Input: part model. Units: mm. Frame: model coordinates. A direction names the side the tool comes from. Round coordinates to 2 decimals unless told otherwise and drop trailing zeros. Loops run counter-clockwise (first coordinate to the right, second up) from the corner with the lowest first, then second, coordinate; pieces in that order, holes last. Notation, with made-up numbers: (-18.75, 15.25) - (27.25, 15.25) arc R24 cw to (27.25, 44.25) - close; hole circle Ø11 at (69.25, -11.75). An arc over 180 degrees is marked (long way). Write each question's results on one line, items separated by ' | '.
from build123d import *

# Parameters (mm, degrees)
THREAD1_PITCH = 1.27


with BuildPart() as part:
    # Sketch1 → Revolve1 (revolve)
    with BuildSketch(Plane.XY, mode=Mode.PRIVATE) as revolve1_sk:
        Polygon((0, 0), (0, 2.9845), (3.81, 2.9845), (3.81, 6.35), (10.16, 6.35), (10.16, 0), align=None)
    revolve(revolve1_sk.sketch.rotate(Axis((10.16, 0, 0), (-1, 0, 0)), 90), axis=Axis((10.16, 0, 0), (-1, 0, 0)))

    # Thread1: the profile of Thread Profile1 profile screwed along a right-hand helix of 3 turns, 8 arcs to a turn; built about Z, then put on its axis
    thread1_z = Axis((0, 0, 0), (0, 0, 1))
    thread1_corners = [(2.9848, 0, -0.000173205), (2.9848, 0, 1.111423202), (2.297092339, 0, 0.714374998), (2.297092339, 0, 0.396874998)]
    with BuildLine(mode=Mode.PRIVATE) as thread1_profile:
        Line(thread1_corners[0], thread1_corners[1])
        Line(thread1_corners[1], thread1_corners[2])
        Line(thread1_corners[2], thread1_corners[3])
        Line(thread1_corners[3], thread1_corners[0])
    thread1_cap = Face(thread1_profile.wire())
    thread1_turn_angles = [0, 22.5, 45, 67.5, 90, 112.5, 135, 157.5, 180, 202.5, 225, 247.5, 270, 292.5, 315, 337.5, 360]
    thread1_turn_weights = [1, 0.9238795325112867, 1, 0.9238795325112867, 1, 0.9238795325112867, 1, 0.9238795325112867, 1, 0.9238795325112867, 1, 0.9238795325112867, 1, 0.9238795325112867, 1, 0.9238795325112867, 1]
    thread1_turn_rails = [Edge.make_bspline([Vector(p[0], p[1], 0).rotate(thread1_z, thread1_turn_angles[k]) / thread1_turn_weights[k] + Vector(0, 0, p[2] + THREAD1_PITCH * thread1_turn_angles[k] / 360) for k in range(17)], [0, 0, 0, 1, 1, 2, 2, 3, 3, 4, 4, 5, 5, 6, 6, 7, 7, 8, 8, 8], 2, thread1_turn_weights) for p in thread1_corners]
    thread1_turn_sides = [Face.make_surface_from_curves(thread1_turn_rails[p[0]], thread1_turn_rails[p[1]]) for p in [(0, 1), (1, 2), (2, 3), (3, 0)]]
    thread1 = Plane(origin=(3.81, 0, 0), x_dir=(0, 0, 1), z_dir=(-1, 0, 0)) * Solid(Shell([*[p.moved(Location((0, 0, THREAD1_PITCH * i))) for i in range(3) for p in thread1_turn_sides], thread1_cap, thread1_cap.rotate(thread1_z, 1080).moved(Location((0, 0, THREAD1_PITCH * 1080 / 360)))]))
    add(thread1, mode=Mode.SUBTRACT)


solid = part.part
1. Section query A-A, the plane x = 9.25. Output: boundary loops of the cut face in (y, z), plus the area to 3 significant figures.
Answer:
outline: circle Ø12.7 at (0, 0) | area: 127 mm^2
2. Section query B-B, the plane z = 4.5. Output: boundary loops of the cut face in (x, y).
Answer:
outline: (3.81, -4.48) - (10.16, -4.48) - (10.16, 4.48) - (3.81, 4.48) - close
3. Line query: line 1 (X direction, y = 0, z = -2.5); line 2 (X direction, y = -1.25, z = 5.5); line 3 (Z direction, x = 9, y = 2.25). Output: solid intervals per line, ascending. Write a range as [from, to].
Answer:
line 1: [0.36, 1.07], [1.63, 2.34], [2.9, 10.16] | line 2: [3.81, 10.16] | line 3: [-5.94, 5.94]
4. Set-up query: faces 1 (the flat face through (3.81, 1, 3)), 2 (the flat face through (0, 0, 0)). Return all of +Z, -Z, +X, -X, +Y, -Y with unobstructed straight access to the full face (end or side cutting, diameter ignored); none if empty.
Answer:
face 1: -X | face 2: +Z, -Z, -X, +Y, -Y
5. Contact query for flat-ended pins moving along their axis: pin 1 (5 mm diameter, centred on x = 7, z = 3.5, fed in from -Y); pin 2 (4 mm diameter, centred on x = 2.5, z = 4, fed in from +Y); pin 3 (6 mm diameter, centred on x = 2, y = 2.5, fed in from +Z). Output: stop coordinate, or through.
Answer:
pin 1: y = -6.27 | pin 2: y = 5.84 | pin 3: z = 6.35
